For this review, take the finished solid that the model builds, in its own axes (mm). A direction names the side the tool comes from. Round coordinates to 2 decimals unless told otherwise and drop trailing zeros. Order: outer loops, then holes, each group sorted by start corner. A loop starts at its lowest first (then second) coordinate and runs counter-clockwise, first axis right, second up. Notation, with made-up numbers: (86, 18.25) - (134, 18.25) arc R11 ccw to (134, 37.25) - close; hole circle Ø9 at (19.25, 44). An arc over 180 degrees is marked (long way). One line per question, with ' | ' between items.
```python
from build123d import *

# Parameters (mm, degrees)
F0_R     = 2.6035
F1_DEPTH = 25.4


with BuildPart() as f1:
    # F0 (on Front) → F1 (new body)
    with BuildSketch(Plane.XZ):
        with BuildLine():
            Line((-4.370089, 12.764578), (-10.618489, 12.764578))
            ThreePointArc((-10.618489, 12.764578), (-12.109211, 12.147101), (-12.726689, 10.656378))
            Line((-12.726689, 10.656378), (-12.726689, 4.407978))
            ThreePointArc((-12.726689, 4.407978), (-11.621789, 3.303078), (-10.516889, 4.407978))
            Line((-10.516889, 4.407978), (-10.516889, 6.464108))
            ThreePointArc((-10.516889, 6.464108), (-9.878719, 7.419196), (-8.752116, 7.195101))
            Line((-8.752116, 7.195101), (-5.465125, 3.90811))
            ThreePointArc((-5.465125, 3.90811), (-4.776871, 2.878066), (-4.535189, 1.663046))
            Line((-4.535189, 1.663046), (-4.535189, -1.533889))
            ThreePointArc((-4.535189, -1.533889), (-4.776871, -2.748909), (-5.465125, -3.778953))
            Line((-5.465125, -3.778953), (-8.752116, -7.065945))
            ThreePointArc((-8.752116, -7.065945), (-9.878719, -7.29004), (-10.516889, -6.334952))
            Line((-10.516889, -6.334952), (-10.516889, -4.278822))
            ThreePointArc((-10.516889, -4.278822), (-11.621789, -3.173922), (-12.726689, -4.278822))
            Line((-12.726689, -4.278822), (-12.726689, -10.527222))
            ThreePointArc((-12.726689, -10.527222), (-12.109211, -12.017944), (-10.618489, -12.635422))
            Line((-10.618489, -12.635422), (-4.370089, -12.635422))
            ThreePointArc((-4.370089, -12.635422), (-3.265189, -11.530522), (-4.370089, -10.425622))
            Line((-4.370089, -10.425622), (-6.426219, -10.425622))
            ThreePointArc((-6.426219, -10.425622), (-7.381307, -9.787452), (-7.157212, -8.660849))
            Line((-7.157212, -8.660849), (-3.87022, -5.373858))
            ThreePointArc((-3.87022, -5.373858), (-2.840176, -4.685604), (-1.625156, -4.443922))
            Line((-1.625156, -4.443922), (1.571779, -4.443922))
            ThreePointArc((1.571779, -4.443922), (2.786799, -4.685604), (3.816843, -5.373858))
            Line((3.816843, -5.373858), (7.103834, -8.660849))
            ThreePointArc((7.103834, -8.660849), (7.327929, -9.787452), (6.372841, -10.425622))
            Line((6.372841, -10.425622), (4.316711, -10.425622))
            ThreePointArc((4.316711, -10.425622), (3.211811, -11.530522), (4.316711, -12.635422))
            Line((4.316711, -12.635422), (10.565111, -12.635422))
            ThreePointArc((10.565111, -12.635422), (12.055834, -12.017944), (12.673311, -10.527222))
            Line((12.673311, -10.527222), (12.673311, -4.278822))
            ThreePointArc((12.673311, -4.278822), (11.568411, -3.173922), (10.463511, -4.278822))
            Line((10.463511, -4.278822), (10.463511, -6.334952))
            ThreePointArc((10.463511, -6.334952), (9.825342, -7.29004), (8.698738, -7.065945))
            Line((8.698738, -7.065945), (5.411747, -3.778953))
            ThreePointArc((5.411747, -3.778953), (4.723494, -2.748909), (4.481811, -1.533889))
            Line((4.481811, -1.533889), (4.481811, 1.663046))
            ThreePointArc((4.481811, 1.663046), (4.723494, 2.878066), (5.411747, 3.90811))
            Line((5.411747, 3.90811), (8.698738, 7.195101))
            ThreePointArc((8.698738, 7.195101), (9.825342, 7.419196), (10.463511, 6.464108))
            Line((10.463511, 6.464108), (10.463511, 4.407978))
            ThreePointArc((10.463511, 4.407978), (11.568411, 3.303078), (12.673311, 4.407978))
            Line((12.673311, 4.407978), (12.673311, 10.656378))
            ThreePointArc((12.673311, 10.656378), (12.055834, 12.147101), (10.565111, 12.764578))
            Line((10.565111, 12.764578), (4.316711, 12.764578))
            ThreePointArc((4.316711, 12.764578), (3.211811, 11.659678), (4.316711, 10.554778))
            Line((4.316711, 10.554778), (6.372841, 10.554778))
            ThreePointArc((6.372841, 10.554778), (7.327929, 9.916609), (7.103834, 8.790005))
            Line((7.103834, 8.790005), (3.816843, 5.503014))
            ThreePointArc((3.816843, 5.503014), (2.786799, 4.814761), (1.571779, 4.573078))
            Line((1.571779, 4.573078), (-1.625156, 4.573078))
            ThreePointArc((-1.625156, 4.573078), (-2.840176, 4.814761), (-3.87022, 5.503014))
            Line((-3.87022, 5.503014), (-7.157212, 8.790005))
            ThreePointArc((-7.157212, 8.790005), (-7.381307, 9.916609), (-6.426219, 10.554778))
            Line((-6.426219, 10.554778), (-4.370089, 10.554778))
            ThreePointArc((-4.370089, 10.554778), (-3.265189, 11.659678), (-4.370089, 12.764578))
        make_face()
        with Locations((-0.026689, 0.064578)):
            Circle(F0_R, mode=Mode.SUBTRACT)
    extrude(amount=F1_DEPTH)


solid = f1.part
```
(1) For faces 4 (the cylindrical face through (-9.894, -12.522, 7.413)), 5 (the flat face through (4.482, -13, 0)), 6 (the flat face through (7, -13, 12.765)), list the 3-axis set-ups (+Z, -Z, +X, -X, +Y, -Y) from which the entire face can be reached by the end or side of a thin tool; tool diameter is ignored.
Output values:
face 4: +Y, -Y | face 5: +X, +Y, -Y | face 6: +Z, +X, -X, +Y, -Y
(2) We need section C-C on x = -6. State the section outline as (y, z) points, plus the area to 3 significant figures.
Output values:
outline: (-25.4, -12.64) - (0, -12.64) - (0, -10.43) - (-25.4, -10.43) - close; (-25.4, -7.5) - (0, -7.5) - (0, -4.31) - (-25.4, -4.31) - close; (-25.4, 4.44) - (0, 4.44) - (0, 7.63) - (-25.4, 7.63) - close; (-25.4, 10.55) - (0, 10.55) - (0, 12.76) - (-25.4, 12.76) - close | area: 274 mm^2
(3) We need section B-B on x = 9.25. State the section outline as (y, z) points, plus the area to 3 significant figures.
Output values:
outline: (-25.4, -12.64) - (0, -12.64) - (0, -7.35) - (-25.4, -7.35) - close; (-25.4, 7.48) - (0, 7.48) - (0, 12.76) - (-25.4, 12.76) - close | area: 268 mm^2
(4) Insertion check: pin 1 (6 mm diameter, centred on x = 0.5, y = -16, fed in from -Z); pin 2 (2.5 mm diameter, centred on x = 0.5, y = -13, fed in from -Z); pin 3 (5 mm diameter, centred on x = 1, y = -18, fed in from +Z). Each pin has a flat end and moves straight along its axis. Give the tip position at first contact, or say it passes through.
Output values:
pin 1: z = -12.27 | pin 2: z = -4.45 | pin 3: z = 12.4
(5) Mouldability with a two-part tool opening along Z and no side actions: class faces 1 (the cylindrical face through (9.8, -12.5, -7.3)), 2 (the flat face through (0, 0, 3)), 3 (the cylindrical face through (12.1, -12.5, 12.1)) as released by +Z, released by -Z, zero draft, split by the parting line, or undercut.
Output values:
face 1: undercut | face 2: zero draft | face 3: released by +Z
(6) We need section A-A on z = 8.25. State the section outline as (x, y) points.
Output values:
outline: (-12.73, -25.4) - (-6.62, -25.4) - (-6.62, 0) - (-12.73, 0) - close; (6.56, -25.4) - (12.67, -25.4) - (12.67, 0) - (6.56, 0) - close
(7) For probe 1 along X at (y, z) = (-10.75, 6); probe 2 along Z at (x, y) = (0, -14); probe 3 along Z at (x, y) = (-5.5, -2), list the stretches that pass through material, from the lowest coordinate up. Write a range as [from, to].
Output values:
probe 1: [-12.73, -10.52], [-7.56, -4.37], [4.31, 7.5], [10.46, 12.67] | probe 2: [-4.44, -2.54], [2.67, 4.57] | probe 3: [-12.64, -10.43], [-7, -3.81], [3.94, 7.13], [10.55, 12.76]
